Verification items for the finished model (mm, model axes). Face numbers are marked on the shaded views. Round coordinates to 2 decimals unless told otherwise and drop trailing zeros. Loops run counter-clockwise (first coordinate to the right, second up) from the corner with the lowest first, then second, coordinate; pieces in that order, holes last. Notation, with made-up numbers: M 80.25,-4 L 117.25,-4 A23 cw 117.25,7 Z; hole C -3.75,62 d8. An arc over 180 degrees is marked long. Answer as CSV lines item,"result".
Autodesk Inventor part; units mm, degrees
ref_plane "YZ Plane" through (0, 0, 0) normal (1, 0, 0) x (0, 1, 0)
ref_plane "XZ Plane" through (0, 0, 0) normal (0, 1, 0) x (-1, 0, 0)
ref_plane "XY Plane" through (0, 0, 0) normal (0, 0, 1) x (1, 0, 0)
sketch "Sketch1" plane through (0, 0, 0) normal (1, 0, 0) x (0, 1, 0)
  point P0 (0, 0)
sketch "Sketch2" plane through (0, 0, 0) normal (1, 0, 0) x (0, 1, 0)
  line L0 (0, 0) -> (25.4, 0)
  line L1 (25.4, 0) -> (25.4, -25.4)
  line L2 (25.4, -25.4) -> (0, -25.4)
  line L3 (0, -25.4) -> (0, 0)
  dimension "d0" = 25.4
  dimension "d1" = 25.4
extrude "Extrusion1" add sketch "Sketch2" along normal blind 101.6
sketch "Sketch3" plane through (101.6, 0, 0) normal (1, 0, 0) x (0, 0, -1)
  line L0 (0, 0) -> (25.4, 0)
  line L1 (0, 0) -> (3.175, 0)
  line L2 (3.175, 0) -> (0, 0)
  line L3 (2.667, 3.175) -> (2.667, 2.5569)
  line L4 (2.667, 2.5569) -> (3.175, 2.5569)
  line L5 (2.667, 2.5569) -> (22.733, 2.5569)
  line L6 (22.733, 2.5569) -> (22.733, 22.837)
  line L7 (22.733, 22.837) -> (2.667, 22.837)
  line L8 (2.667, 22.837) -> (2.667, 2.5569)
extrude "Extrusion2" cut sketch "Sketch3" against normal blind 50.8
sketch "Sketch4" plane through (0, 0, 0) normal (-1, 0, 0) x (0, 0, 1)
  line L0 (-25.4, 0) -> (-25.4, 25.4)
  line L1 (-25.4, 25.4) -> (0, 25.4)
  line L2 (-22.225, 3.175) -> (-3.175, 3.175)
  line L3 (-22.225, 22.225) -> (-22.225, 3.175)
  line L4 (-21.59, 3.302) -> (-22.098, 3.302)
  line L5 (-17.272, 8.128) -> (-8.128, 8.128)
  line L6 (-8.128, 8.128) -> (-8.128, 17.907)
  line L7 (-8.128, 17.907) -> (-17.272, 17.907)
  line L8 (-17.272, 17.907) -> (-17.272, 8.128)
  line L9 (-22.098, 3.302) -> (-3.302, 3.302)
  line L10 (-3.302, 3.302) -> (-3.302, 22.733)
  line L11 (-3.302, 22.733) -> (-22.098, 22.733)
  line L12 (-22.098, 22.733) -> (-22.098, 3.302)
extrude "Extrusion3" cut sketch "Sketch4" against normal blind 38.1
properties part number "Left Side Piece Corrected 0.02 inch"
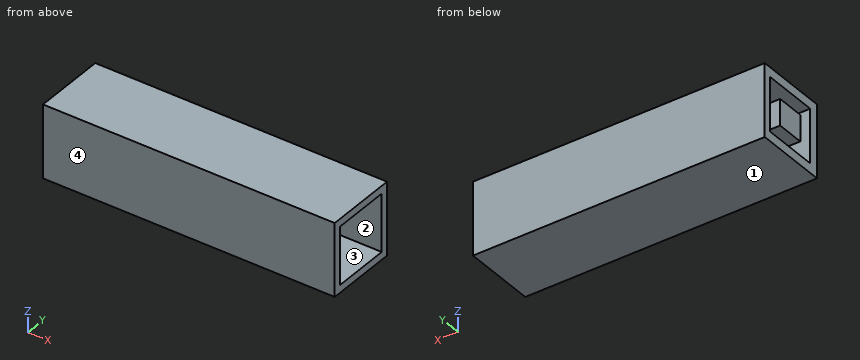
1) Section check C-C (z = -4.5). Record the cut outline in (x, y), plus the area to 3 significant figures.
Here are the results:
outline,"M 0,0 L 101.6,0 L 101.6,2.56 L 50.8,2.56 L 50.8,22.84 L 101.6,22.84 L 101.6,25.4 L 0,25.4 L 0,22.73 L 38.1,22.73 L 38.1,3.3 L 0,3.3 Z"
area,"810 mm^2"
2) Section check D-D (x = 89). Record the cut outline in (y, z), plus the area to 3 significant figures.
Here are the results:
outline,"M 0,-25.4 L 25.4,-25.4 L 25.4,0 L 0,0 Z; hole M 2.56,-22.73 L 22.84,-22.73 L 22.84,-2.67 L 2.56,-2.67 Z"
area,"238 mm^2"
3) Section check B-B (y = 20.75). Record the cut outline in (x, z).
Here are the results:
outline,"M 0,-25.4 L 101.6,-25.4 L 101.6,-22.73 L 50.8,-22.73 L 50.8,-2.67 L 101.6,-2.67 L 101.6,0 L 0,0 L 0,-3.3 L 38.1,-3.3 L 38.1,-22.1 L 0,-22.1 Z"
4) Go/stop test with flat-tipped pins: pin 1 (2 mm diameter, centred on y = 12, z = -14, fed in from +X); pin 2 (2 mm diameter, centred on x = 26, y = 12.5, fed in from +Z). Record where each tip stops, or that it passes through.
Here are the results:
pin 1,"stops at x = 50.8"
pin 2,"stops at z = 0"
5) Draft check along Y on the marked faces 1, 2, 3 and 4. Enter one of: +Y half, -Y half, draft (parallel to the pull), parting line (faces both ways), or undercut.
Here are the results:
face 1,"draft"
face 2,"undercut"
face 3,"undercut"
face 4,"-Y half"
6) Section check A-A (x = 24.5). Record the cut outline in (y, z), plus the area to 3 significant figures.
Here are the results:
outline,"M 0,-25.4 L 25.4,-25.4 L 25.4,0 L 0,0 Z; M 8.13,-17.27 L 17.91,-17.27 L 17.91,-8.13 L 8.13,-8.13 Z; hole M 3.3,-22.1 L 22.73,-22.1 L 22.73,-3.3 L 3.3,-3.3 Z"
area,"369 mm^2"
7) Material ranges on probe 1 along Z at (x, y) = (28, 13); probe 2 along Y at (x, z) = (89, -10.25); probe 3 along Y at (x, z) = (36, -6.5), recorded low to high.
Here are the results:
probe 1,"z = -25.4 to -22.1, -17.27 to -8.13, -3.3 to 0"
probe 2,"y = 0 to 2.56, 22.84 to 25.4"
probe 3,"y = 0 to 3.3, 22.73 to 25.4"
